Build history of the part. All positions in model axes, mm. Give positions to 0.01 mm unless a question says otherwise; leave off trailing zeros. Write each loop counter-clockwise with the first axis right and the second up, starting at its lowest first coordinate (ties: lowest second). Pieces come first, ordered by that corner, then holes. Notation, with made-up numbers: (-31.5, -22) -> (-21.5, -22) arc R20 ccw to (-21.5, -13) -> close; hole circle Ø8 at (55.25, -31.75). An arc over 180 degrees is marked (long way). Put each result on its own line as item: value. Start each with the question number.
Item 1: Slice it at A-A, the plane x = 74. List the corners of the cut face in (y, z), plus the area to 3 significant figures.
Item 2: Flat gauge pin, fed straight in: pin 1 Ø1 at (y, z) = (5, -26.5) entering from +X. Where does the tip first touch, or does it go through?
Item 3: Drill centre lines: line 1 along X through (y, z) = (2, -42.5); line 2 along Z through (x, y) = (17.5, 1); line 3 along X through (y, z) = (2.5, -43). Where is each one in solid material? Low to high.
Item 4: Slice it at B-B, the plane z = -22. List the corners of the cut face in (x, y).
```python
from build123d import *

# Parameters (mm, degrees)
BOSS_EXTRUDE2_DEPTH = 6.35


with BuildPart() as part:
    # Sketch1 → Boss-Extrude2 (new body)
    # profile 1 of 5: a face of its own
    with BuildSketch(Plane(origin=(0, 0, 0), x_dir=(1, 0, 0), z_dir=(0, 1, 0))):
        with BuildLine():
            Line((19.05, 45.006744084), (19.05, 59.294244084))
            ThreePointArc((19.05, 59.294244084), (5.579615818, 53.714628266), (0, 40.244244084))
            Line((0, 40.244244084), (0, 0))
            Line((0, 0), (19.05, 0))
            Line((19.05, 0), (19.05, 8.89))
            Line((19.05, 8.89), (8.89, 8.89))
            Line((8.89, 8.89), (8.89, 24.129750608))
            ThreePointArc((8.89, 24.129750608), (13.762212217, 21.942828828), (19.05, 21.194244084))
            Line((19.05, 21.194244084), (19.05, 35.481744084))
            ThreePointArc((19.05, 35.481744084), (14.2875, 40.244244084), (19.05, 45.006744084))
        make_face()
    # profile 2 of 5: a face of its own
    with BuildSketch(Plane(origin=(0, 0, 0), x_dir=(1, 0, 0), z_dir=(0, 1, 0))):
        with BuildLine():
            ThreePointArc((29.976631112, 55.849090528), (24.778445481, 58.412551996), (19.05, 59.294244084))
            Line((19.05, 59.294244084), (19.05, 45.006744084))
            ThreePointArc((19.05, 45.006744084), (22.417596045, 43.611840129), (23.8125, 40.244244084))
            ThreePointArc((23.8125, 40.244244084), (22.417596045, 36.876648039), (19.05, 35.481744084))
            Line((19.05, 35.481744084), (19.05, 21.194244084))
            ThreePointArc((19.05, 21.194244084), (22.242798897, 21.463708011), (25.345272951, 22.264476608))
            Line((25.345272951, 22.264476608), (34.29, 8.89))
            Line((34.29, 8.89), (19.05, 8.89))
            Line((19.05, 8.89), (19.05, 0))
            Line((19.05, 0), (109.737398428, 0))
            Line((109.737398428, 0), (29.976631112, 55.849090528))
        make_face()
        with BuildLine():
            Line((46.99, 8.89), (33.57249636, 27.915432321))
            ThreePointArc((33.57249636, 27.915432321), (35.515172131, 30.66298077), (36.94411395, 33.709476611))
            Line((36.94411395, 33.709476611), (72.39, 8.89))
            Line((72.39, 8.89), (46.99, 8.89))
        make_face(mode=Mode.SUBTRACT)
    # profile 3 of 5: a face of its own
    with BuildSketch(Plane(origin=(0, 0, 0), x_dir=(1, 0, 0), z_dir=(0, 1, 0))):
        with BuildLine():
            ThreePointArc((25.345272951, 22.264476608), (22.242798897, 21.463708011), (19.05, 21.194244084))
            Line((19.05, 21.194244084), (19.05, 8.89))
            Line((19.05, 8.89), (34.29, 8.89))
            Line((34.29, 8.89), (25.345272951, 22.264476608))
        make_face()
    # profile 4 of 5: a face of its own
    with BuildSketch(Plane(origin=(0, 0, 0), x_dir=(1, 0, 0), z_dir=(0, 1, 0))):
        with BuildLine():
            Line((19.05, 8.89), (19.05, 21.194244084))
            ThreePointArc((19.05, 21.194244084), (13.762212217, 21.942828828), (8.89, 24.129750608))
            Line((8.89, 24.129750608), (8.89, 8.89))
            Line((8.89, 8.89), (19.05, 8.89))
        make_face()
    # profile 5 of 5: a face of its own
    with BuildSketch(Plane(origin=(0, 0, 0), x_dir=(1, 0, 0), z_dir=(0, 1, 0))):
        with BuildLine():
            ThreePointArc((33.57249636, 27.915432321), (35.515172131, 30.66298077), (36.94411395, 33.709476611))
            Line((36.94411395, 33.709476611), (72.39, 8.89))
            Line((72.39, 8.89), (46.99, 8.89))
            Line((46.99, 8.89), (33.57249636, 27.915432321))
        make_face()
    extrude(amount=BOSS_EXTRUDE2_DEPTH)


solid = part.part
```
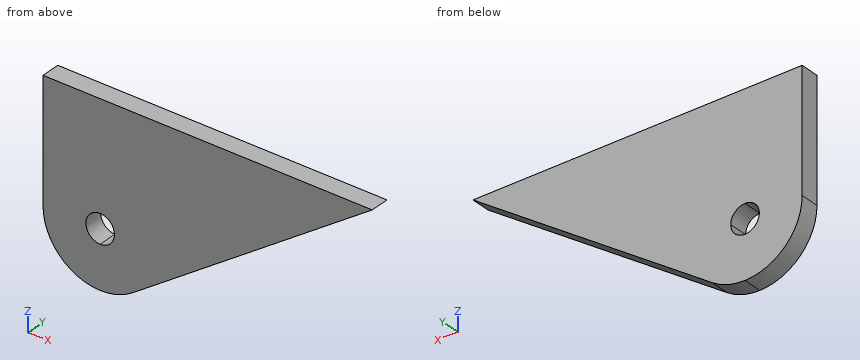
Values follow:
1. outline: (0, -25.02) -> (6.35, -25.02) -> (6.35, 0) -> (0, 0) -> close
1. area: 159 mm2
2. pin 1: x = 72.61
3. line 1: 0.13 to 14.86, 23.24 to 49.04
3. line 2: -59.23 to -44.75, -35.74 to 0
3. line 3: 0.2 to 15.17, 22.93 to 48.33
4. outline: (0, 0) -> (78.32, 0) -> (78.32, 6.35) -> (0, 6.35) -> close
